from build123d import *

# Parameters (mm, degrees)
BOSS_EXTRUDE1_DEPTH = 12.7
BOSS_EXTRUDE2_START = -38.1
SKETCH2_R           = 38.1
SKETCH2_R_2         = 28.575
BOSS_EXTRUDE2_DEPTH = 38.1
CUT_EXTRUDE1_DEPTH  = 38.1


with BuildPart() as part:
    # Sketch1 → Boss-Extrude1 (new body)
    with BuildSketch(Plane(origin=(0, 0, 0), x_dir=(0, 0, -1), z_dir=(1, 0, 0))):
        with BuildLine():
            ThreePointArc((3.175, 28.398063314), (0, 28.575), (-3.175, 28.398063314))
            Line((-3.175, 28.398063314), (-3.175, 12.296722124))
            ThreePointArc((-3.175, 12.296722124), (-10.998522628, 6.35), (-12.236773743, -3.398730405))
            Line((-12.236773743, -3.398730405), (-26.180944248, -11.449401))
            ThreePointArc((-26.180944248, -11.449401), (-24.746675913, -14.2875), (-23.005944248, -16.948662314))
            Line((-23.005944248, -16.948662314), (-9.061773743, -8.897991719))
            ThreePointArc((-9.061773743, -8.897991719), (0, -12.7), (9.061773743, -8.897991719))
            Line((9.061773743, -8.897991719), (23.005944248, -16.948662314))
            ThreePointArc((23.005944248, -16.948662314), (24.746675913, -14.2875), (26.180944248, -11.449401))
            Line((26.180944248, -11.449401), (12.236773743, -3.398730405))
            ThreePointArc((12.236773743, -3.398730405), (10.998522628, 6.35), (3.175, 12.296722124))
            Line((3.175, 12.296722124), (3.175, 28.398063314))
        make_face()
    extrude(amount=BOSS_EXTRUDE1_DEPTH)

    # Sketch2 → Boss-Extrude2 (add)
    with BuildSketch(Plane(origin=(25.4, 0, 0), x_dir=(0, 0, -1), z_dir=(1, 0, 0)).offset(BOSS_EXTRUDE2_START)):
        Circle(SKETCH2_R)
        Circle(SKETCH2_R_2, mode=Mode.SUBTRACT)
    extrude(amount=BOSS_EXTRUDE2_DEPTH)

    # Sketch3 → Cut-Extrude1 (cut)
    with BuildSketch(Plane(origin=(12.7, 0, 0), x_dir=(0, 0, -1), z_dir=(1, 0, 0))):
        Polygon((0, 7.332348419), (-6.35, 3.666174209), (-6.35, -3.666174209), (0, -7.332348419), (6.35, -3.666174209), (6.35, 3.666174209), align=None)
    extrude(amount=-CUT_EXTRUDE1_DEPTH, mode=Mode.SUBTRACT)


solid = part.part
Verification items for the finished model (mm, model axes). A direction names the side the tool comes from. Coordinates: 2 decimals unless noted, no trailing zeros. Order: outer loops, then holes, each group sorted by start corner. A loop starts at its lowest first (then second) coordinate and runs counter-clockwise, first axis right, second up. Notation, with made-up numbers: M -32,57.25 L 12,57.25 A18 cw 12,81.25 Z; hole C -5,8.25 d11. An arc over 180 degrees is marked long. One line per item, written item: value. Start each with the question number.
Item 1: Mould release check, pull along Y, two halves, no side actions. Record for faces 1 (the cylindrical face through (6.083, -23.183, 30.235)), 2 (the flat face through (25.4, 28.4, -5.5)), 3 (the flat face through (6.26, -12.87, -15.94)): pulls with the +Y half, pulls with the -Y half, needs draft (parallel to the pull), parting line crosses it, or undercut.
Item 2: Sectioned sample at D-D on y = 0. Record the cut outline in (x, z) (3 decimals), then the cut area to 3 significant figures.
Item 3: Depth check by flat-ended pin: P1, Ø8, axis at x = -1.5, z = -20.5, coming from the +Y side; P2, Ø1, axis at x = 10, z = -10, coming from the -Y side; P3, Ø14, axis at x = 5, y = 22, coming from the +Z side; P4, Ø3, axis at y = -2, z = -26, coming from the +X side. Enter the tip coordinate at first touch or a pass-through.
Item 4: Sectioned sample at B-B on y = 18. Record the cut outline in (x, z) (3 decimals), then the cut area to 3 significant figures.
Item 5: Sectioned sample at C-C on z = -10.5. Record the cut outline in (x, y), then the cut area to 3 significant figures.
Item 6: Access from +Z, -Z, +X, -X, +Y, -Y to the whole of each face (thin tool, end or side, straight path). Record for faces 4 (the flat face through (-12.7, 28.4, -5.5)), 5 (the flat face through (0, -6, 4)), 6 (the flat face through (6.261, -7.368, 19.111)).
Item 7: Thickness scan on probe 1 along Y at (x, z) = (12.5, 0) (3 decimals); probe 2 along Y at (x, z) = (-4, 0) (3 decimals); probe 3 along Y at (x, z) = (8, 5). Record the ranges inside material, lowest first.
Item 8: Sectioned sample at A-A on x = 3. Record the cut outline in (y, z) (3 decimals).
Calculated:
1. face 1: parting line crosses it
1. face 2: needs draft
1. face 3: undercut
2. outline: M -12.7,-38.1 L 25.4,-38.1 L 25.4,-28.575 L -12.7,-28.575 Z; M -12.7,28.575 L 25.4,28.575 L 25.4,38.1 L -12.7,38.1 Z; M 0,-12.7 L 12.7,-12.7 L 12.7,-6.35 L 0,-6.35 Z; M 0,6.35 L 12.7,6.35 L 12.7,12.7 L 0,12.7 Z
2. area: 887 mm^2
3. P1: y = 34.34
3. P2: y = -36.9
3. P3: z = 35.02
3. P4: through
4. outline: M -12.7,-33.58 L 25.4,-33.58 L 25.4,-22.193 L -12.7,-22.193 Z; M -12.7,22.193 L 25.4,22.193 L 25.4,33.58 L -12.7,33.58 Z; M 0,-3.175 L 12.7,-3.175 L 12.7,3.175 L 0,3.175 Z
4. area: 948 mm^2
5. outline: M -12.7,-36.62 L 25.4,-36.62 L 25.4,-26.58 L -12.7,-26.58 Z; M -12.7,26.58 L 25.4,26.58 L 25.4,36.62 L -12.7,36.62 Z; M 0,-9.73 L 12.7,-9.73 L 12.7,7.14 L 0,7.14 Z
5. area: 980 mm^2
6. face 4: +Z, -Z, -X, +Y, -Y
6. face 5: -X
6. face 6: +X, -X
7. probe 1: -38.1 to -28.575, -12.7 to -7.332, 7.332 to 38.1
7. probe 2: -38.1 to -28.575, 28.575 to 38.1
7. probe 3: -37.77 to -28.13, -11.67 to -4.45, 4.45 to 11.67, 28.13 to 37.77
8. outline: C 0,0 d76.2; hole M -16.949,-23.006 L -8.898,-9.062 A12.7 cw -8.898,9.062 L -16.949,23.006 A28.575 ccw Z; hole M -11.449,-26.181 A28.575 ccw 28.398,-3.175 L 12.297,-3.175 A12.7 cw -3.399,-12.237 Z; hole M -11.449,26.181 L -3.399,12.237 A12.7 cw 12.297,3.175 L 28.398,3.175 A28.575 ccw Z; hole M -7.332,0 L -3.666,-6.35 L 3.666,-6.35 L 7.332,0 L 3.666,6.35 L -3.666,6.35 Z
